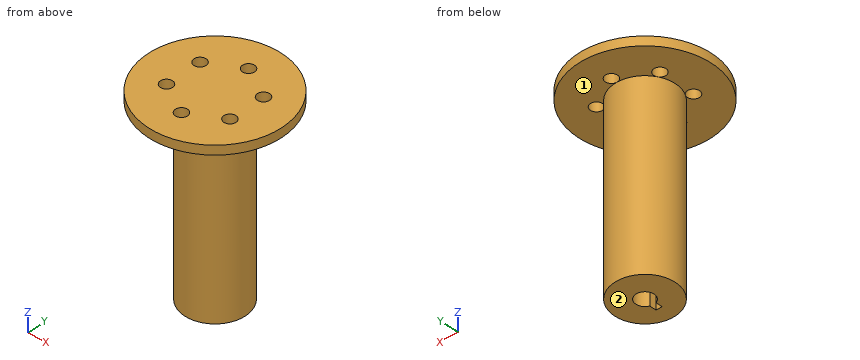
```python
from build123d import *

# Parameters (mm, degrees)
SKETCH1_R           = 5
BOSS_EXTRUDE1_DEPTH = 30
CUT_EXTRUDE1_DEPTH  = 20
SKETCH3_R           = 11
BOSS_EXTRUDE2_DEPTH = 1.5
SKETCH4_R           = 1
CUT_EXTRUDE2_DEPTH  = 1.5


with BuildPart() as part:
    # Sketch1 → Boss-Extrude1 (new body)
    with BuildSketch(Plane.XY):
        Circle(SKETCH1_R)
    extrude(amount=BOSS_EXTRUDE1_DEPTH)

    # Sketch2 → Cut-Extrude1 (cut)
    with BuildSketch(Plane(origin=(0, 0, 0), x_dir=(-1, 0, 0), z_dir=(0, 0, -1))):
        with BuildLine():
            Line((-0.5, -1.414213562), (-0.5, -2.514037514))
            Line((-0.5, -2.514037514), (0.5, -2.514037514))
            Line((0.5, -2.514037514), (0.5, -1.414213562))
            ThreePointArc((0.5, -1.414213562), (0, 1.5), (-0.5, -1.414213562))
        make_face()
    extrude(amount=-CUT_EXTRUDE1_DEPTH, mode=Mode.SUBTRACT)

    # Sketch3 → Boss-Extrude2 (add)
    with BuildSketch(Plane.XY.offset(30)):
        Circle(SKETCH3_R)
    extrude(amount=BOSS_EXTRUDE2_DEPTH)

    # Sketch4 → Cut-Extrude2 (cut)
    with BuildSketch(Plane.XY.offset(31.5)):
        with Locations((0, 6)):
            Circle(SKETCH4_R)
        with Locations((5.196152423, 3)):
            Circle(SKETCH4_R)
        with Locations((5.196152423, -3)):
            Circle(SKETCH4_R)
        with Locations((0, -6)):
            Circle(SKETCH4_R)
        with Locations((-5.196152423, -3)):
            Circle(SKETCH4_R)
        with Locations((-5.196152423, 3)):
            Circle(SKETCH4_R)
    extrude(amount=-CUT_EXTRUDE2_DEPTH, mode=Mode.SUBTRACT)


solid = part.part
```
Design review of the part built by this model. Coordinates are the model's own, in mm. Face numbers are marked on the shaded views. A direction names the side the tool comes from. Give positions to 0.01 mm unless a question says otherwise; leave off trailing zeros. Loops run counter-clockwise (first coordinate to the right, second up) from the corner with the lowest first, then second, coordinate; pieces in that order, holes last. Notation, with made-up numbers: (-30.75, 57.5) -> (-5.75, 57.5) arc R30 ccw to (-5.75, 89.5) -> close; hole circle Ø4 at (83, -35). An arc over 180 degrees is marked (long way). Write each question's results on one line, items separated by ' | '.
Q1. Machinability: for the marked faces 1 and 2, which of the approach directions +Z, -Z, +X, -X, +Y, -Y give a long, thin tool a straight path to every point of the face, cutting with its end or side? Answer none if there is none.
Reply:
face 1: -Z | face 2: -Z, +X, -X, +Y, -Y
Q2. Take a section at B-B, the plane z = 5.5. Write out the cut boundary in (x, y), plus the area to 3 significant figures.
Reply:
outline: circle Ø10 at (0, 0); hole (-0.5, -2.51) -> (0.5, -2.51) -> (0.5, -1.41) arc R1.5 ccw (long way) to (-0.5, -1.41) -> close | area: 70.4 mm²
Q3. Take a section at D-D, the plane y = -6. Write out the cut boundary in (x, z).
Reply:
outline: (-9.22, 30) -> (-1, 30) -> (-1, 31.5) -> (-9.22, 31.5) -> close; (1, 30) -> (9.22, 30) -> (9.22, 31.5) -> (1, 31.5) -> close
Q4. Take a section at A-A, the plane y = 0. Write out the cut boundary in (x, z).
Reply:
outline: (-11, 30) -> (-5, 30) -> (-5, 0) -> (-1.5, 0) -> (-1.5, 20) -> (1.5, 20) -> (1.5, 0) -> (5, 0) -> (5, 30) -> (11, 30) -> (11, 31.5) -> (-11, 31.5) -> close
Q5. Take a section at C-C, the plane x = 2. Write out the cut boundary in (y, z).
Reply:
outline: (-10.82, 30) -> (-4.58, 30) -> (-4.58, 0) -> (4.58, 0) -> (4.58, 30) -> (10.82, 30) -> (10.82, 31.5) -> (-10.82, 31.5) -> close
Q6. For pin 1 Ø2.5 at (x, y) = (-5.2, -3) entering from -Z; pin 2 Ø1.5 at (x, y) = (0.5, -0.5) entering from -Z; pin 3 Ø0.9 at (y, z) = (-2, 9) entering from -X; pin 4 Ø12 at (x, z) = (0, 5.5) entering from +Y, all flat-tipped, find the tip position at first contact; note any pin that passes through.
Reply:
pin 1: stops at z = 0 | pin 2: stops at z = 20 | pin 3: stops at x = -4.75 | pin 4: stops at y = 5
Q7. Wall thickness on L1, parallel to Y at x = 0, z = 30.95; L2, parallel to X at y = -3, z = 30.95; L3, parallel to Y at x = 6, z = 30.5: over which ranges is each line inside the solid? List them lowest first.
Reply:
L1: y = -11 to -7, -5 to 5, 7 to 11 | L2: x = -10.58 to -6.2, -4.2 to 4.2, 6.2 to 10.58 | L3: y = -9.22 to -3.59, -2.41 to 2.41, 3.59 to 9.22
